from build123d import *

# Parameters (mm, degrees)
BOSS_EXTRUDE1_DEPTH           = 7
BOSS_EXTRUDE1_TAPER           = 37
BOSS_EXTRUDE1_OTHER_WAY_DEPTH = 5
SKETCH2_R                     = 1.75
CUT_EXTRUDE1_DEPTH            = 3
SKETCH3_R                     = 79.208746666
BOSS_EXTRUDE2_DEPTH           = 10
MIRROR1_START                 = -64.52
MIRROR1_DEPTH                 = 5


with BuildPart() as part:
    # Sketch1 → Boss-Extrude1 (new body)
    with BuildSketch(Plane.XY):
        Polygon((-10, 101.234331062), (-59.142135624, 14.142135624), (-45, 0), (45, 0), (59.142135624, 14.142135624), (10, 101.234331062), align=None)
    extrude(amount=BOSS_EXTRUDE1_DEPTH, taper=BOSS_EXTRUDE1_TAPER)

    # Sketch1 → Boss-Extrude1 other way (add)
    with BuildSketch(Plane.XY):
        Polygon((-10, 101.234331062), (-59.142135624, 14.142135624), (-45, 0), (45, 0), (59.142135624, 14.142135624), (10, 101.234331062), align=None)
    extrude(amount=-BOSS_EXTRUDE1_OTHER_WAY_DEPTH)

    # Sketch2 → Cut-Extrude1 (cut)
    with BuildSketch(Plane(origin=(0, 0, -5), x_dir=(-1, 0, 0), z_dir=(0, 0, -1))):
        with Locations((0, 81.234331062)):
            Circle(SKETCH2_R)
    extrude(amount=-CUT_EXTRUDE1_DEPTH, mode=Mode.SUBTRACT)

    # Sketch3 → Boss-Extrude2 (add)
    with BuildSketch(Plane.XZ):
        with Locations((0, -32.26)):
            Circle(SKETCH3_R)
    extrude(amount=BOSS_EXTRUDE2_DEPTH)

    # Mirror1: read off the stored shape, not the designer's step
    # Mirror1 outline → Mirror1 (add)
    with BuildSketch(Plane.XY.offset(MIRROR1_START)):
        Polygon((-10, 101.234331062), (-59.142135624, 14.142135624), (-45, 0), (45, 0), (59.142135624, 14.142135624), (10, 101.234331062), align=None)
    extrude(amount=MIRROR1_DEPTH)

    # Mirror1 2: loft between two sections, ruled curve by curve
    mirror1_2_from = [
        Edge.make_line((-10, 101.234331062, -64.52), (-59.142135624, 14.142135624, -64.52)),
        Edge.make_line((10, 101.234331062, -64.52), (-10, 101.234331062, -64.52)),
        Edge.make_line((59.142135624, 14.142135624, -64.52), (10, 101.234331062, -64.52)),
        Edge.make_line((45, 0, -64.52), (59.142135624, 14.142135624, -64.52)),
        Edge.make_line((-45, 0, -64.52), (45, 0, -64.52)),
        Edge.make_line((-59.142135624, 14.142135624, -64.52), (-45, 0, -64.52)),
    ]
    mirror1_2_to = [
        Edge.make_line((-6.919711963, 95.959452712, -71.52), (-52.579336418, 15.039140921, -71.52)),
        Edge.make_line((6.919711963, 95.959452712, -71.52), (-6.919711963, 95.959452712, -71.52)),
        Edge.make_line((52.579336418, 15.039140921, -71.52), (6.919711963, 95.959452712, -71.52)),
        Edge.make_line((42.815073847, 5.274878351, -71.52), (52.579336418, 15.039140921, -71.52)),
        Edge.make_line((-42.815073847, 5.274878351, -71.52), (42.815073847, 5.274878351, -71.52)),
        Edge.make_line((-52.579336418, 15.039140921, -71.52), (-42.815073847, 5.274878351, -71.52)),
    ]
    mirror1_2 = Solid(Shell([*[Face.make_surface_from_curves(mirror1_2_from[k], mirror1_2_to[k]) for k in range(6)], Face(Wire(mirror1_2_from)), Face(Wire(mirror1_2_to))]))
    add(mirror1_2)


solid = part.part
Can you work these out from the model? Positions are in its coordinate system, mm. A direction names the side the tool comes from. Round coordinates to 2 decimals unless told otherwise and drop trailing zeros. Order: outer loops, then holes, each group sorted by start corner. A loop starts at its lowest first (then second) coordinate and runs counter-clockwise, first axis right, second up. Notation, with made-up numbers: (73, -18) - (130, -18) arc R12 cw to (130, -2) - close; hole circle Ø4 at (31.25, 23.25). An arc over 180 degrees is marked (long way). Answer in a Markdown table with one row per item.
(1) Please list where these lines run through material, in increasing order: L1, parallel to Z at x = -27, y = 28; L2, parallel to Y at x = 0, z = -3.25; L3, parallel to Y at x = -15, z = -90. Write a range as from..to.
From the geometry:
| item | result |
|---|---|
| L1 | z = -71.52..-59.52, -5..7 |
| L2 | y = -10..79.48, 82.98..101.23 |
| L3 | y = -10..0 |
(2) For P1, Ø3, axis at x = -0.5, y = 80.5, coming from the -Z side; P2, Ø12, axis at y = 42, z = -69.5, coming from the +X side; P3, Ø3, axis at x = 0, y = 81.23, coming from the +Z side, each with a flat end and sliding along its axis, tell me the tip position at first contact or that it passes through.
From the geometry:
| item | result |
|---|---|
| P1 | stops at z = -71.52 |
| P2 | stops at x = 45.31 |
| P3 | stops at z = 7 |
(3) If we mould it in two halves opening along Y, with no side actions, what happens to faces 1 (the face through (0, 101.234, -62)), 2 (the face through (-52, 7, -62)), 3 (the face through (-62.857, -4.93, -80.457))? For each: released by +Y, released by -Y, zero draft, split by the parting line, or undercut.
From the geometry:
| item | result |
|---|---|
| face 1 | released by +Y |
| face 2 | undercut |
| face 3 | zero draft |
(4) Suppose I cut it at A-A, the plane z = -32.26. Please give me the cut outline in (x, y), plus the area to 3 significant figures.
From the geometry:
| item | result |
|---|---|
| outline | (-79.21, -10) - (79.21, -10) - (79.21, 0) - (-79.21, 0) - close |
| area | 1,580 mm2 |
(5) Which directions (+Z, -Z, +X, -X, +Y, -Y) give clear straight access to the entire face, cutting with the end or side of a thin tool? Please do faces 4 (the face through (-1, 41, -71.52)), 5 (the face through (-1, 40, -59.52)), 6 (the face through (52, 7, -2)), 7 (the face through (-50.13, 8.81, 3.45)).
From the geometry:
| item | result |
|---|---|
| face 4 | -Z, +X, -X, +Y |
| face 5 | +X, -X, +Y |
| face 6 | +Z, -Z, +X |
| face 7 | +Z, -X |
(6) Suppose I cut it at B-B, the plane z = 28.5. Please give me the cut outline in (x, y).
From the geometry:
| item | result |
|---|---|
| outline | (-50.82, -10) - (50.82, -10) - (50.82, 0) - (-50.82, 0) - close |
